Autodesk Inventor part; units mm, degrees
ref_plane "YZ Plane" through (0, 0, 0) normal (1, 0, 0) x (0, 1, 0)
ref_plane "XZ Plane" through (0, 0, 0) normal (0, 1, 0) x (-1, 0, 0)
ref_plane "XY Plane" through (0, 0, 0) normal (0, 0, 1) x (1, 0, 0)
sketch "Sketch1" plane through (0, 0, 0) normal (0, 1, 0) x (-1, 0, 0)
  line L0 (0, 0) -> (50, 0)
  line L1 (50, 0) -> (50, -70)
  line L2 (50, -70) -> (0, -70)
  line L3 (0, -70) -> (0, 0)
  dimension "d0" = 50
  dimension "d1" = 70
extrude "Extrusion1" add sketch "Sketch1" along normal blind 2
sketch "Sketch2" plane through (0, 2, 0) normal (0, 1, 0) x (1, 0, 0)
  line L0 (-47.6458, 6.5409) -> (-28.6458, 6.5409)
  line L1 (-28.6458, 6.5409) -> (-28.6458, 18.5409)
  line L2 (-28.6458, 18.5409) -> (-47.6458, 18.5409)
  line L3 (-47.6458, 18.5409) -> (-47.6458, 6.5409)
  line L4 (-47.6458, 26.8862) -> (-28.6458, 26.8862)
  line L5 (-28.6458, 26.8862) -> (-28.6458, 38.8862)
  line L6 (-28.6458, 38.8862) -> (-47.6458, 38.8862)
  line L7 (-47.6458, 38.8862) -> (-47.6458, 26.8862)
  line L8 (-47.6458, 47.2315) -> (-28.6458, 47.2315)
  line L9 (-28.6458, 47.2315) -> (-28.6458, 59.2315)
  line L10 (-28.6458, 59.2315) -> (-47.6458, 59.2315)
  line L11 (-47.6458, 59.2315) -> (-47.6458, 47.2315)
  point P0 (0, 0)
  dimension "d4" = 19
  dimension "d5" = 12
  dimension "d6" = 19
  dimension "d7" = 12
  dimension "d8" = 19
  dimension "d9" = 12
extrude "Extrusion2" add sketch "Sketch2" along normal blind 20
properties part number "temp_pcb"
Geometry check sheet. Reference: the model listing, model coordinates, mm. A direction names the side the tool comes from. Give positions to 0.01 mm unless a question says otherwise; leave off trailing zeros. Loops run counter-clockwise (first coordinate to the right, second up) from the corner with the lowest first, then second, coordinate; pieces in that order, holes last. Notation, with made-up numbers: (-3.75, 73.25) -> (37.25, 73.25) arc R22 ccw to (37.25, 80.25) -> close; hole circle Ø7 at (38.25, 71.5). An arc over 180 degrees is marked (long way). Answer in a Markdown table with one row per item. Add a question column.
1) Cross-section at C-C on x = -42. Record the boundary of the cut face in (y, z).
2) Gauge pin test, flat ends, axial feed: P1, Ø9.5, axis at y = 13, z = -53.5, coming from the -X side; P2, Ø9.5, axis at x = -38, y = 8, coming from the +Z side; P3, Ø15, axis at x = -16.5, z = -43.5, coming from the +Y side; P4, Ø10, axis at x = -19, y = 10.5, coming from the +Z side. Record the tip position at first contact, or that the pin passes through.
3) Cross-section at B-B on z = -8. Record the boundary of the cut face in (x, y), and give its area (3 significant figures).
4) Material ranges on probe 1 along Z at (x, y) = (-44, 8.25); probe 2 along Y at (x, z) = (-7, -43); probe 3 along X at (y, z) = (20.5, -58), recorded low to high. Write a range as from..to.
5) Cross-section at A-A on y = 8.5. Record the boundary of the cut face in (x, z), and give its area (3 significant figures).
6) Draft check along Z on faces 1 (the face through (-38, 12, -18.541)), 2 (the face through (-38, 12, -6.541)), 3 (the face through (-28.646, 12, -53)). Enter one of: pulls with the +Z half, pulls with the -Z half, needs draft (parallel to the pull), parting line crosses it, or undercut.
7) Cross-section at D-D on z = -66. Record the boundary of the cut face in (x, y), and give its area (3 significant figures).
8) Set-up check for faces 4 (the face through (-38, 12, -38.886)), 5 (the face through (-38, 12, -59.232)), 6 (the face through (-47.646, 12, -13)): record each of +Z, -Z, +X, -X, +Y, -Y from which the full face is reachable in a straight line by a thin tool's end or side.
Outcome:
| question | item | result |
|---|---|---|
| 1 | outline | (0, -70) -> (2, -70) -> (2, -59.23) -> (22, -59.23) -> (22, -47.23) -> (2, -47.23) -> (2, -38.89) -> (22, -38.89) -> (22, -26.89) -> (2, -26.89) -> (2, -18.54) -> (22, -18.54) -> (22, -6.54) -> (2, -6.54) -> (2, 0) -> (0, 0) -> close |
| 2 | P1 | stops at x = -47.65 |
| 2 | P2 | stops at z = -6.54 |
| 2 | P3 | stops at y = 2 |
| 2 | P4 | passes through |
| 3 | outline | (-50, 0) -> (0, 0) -> (0, 2) -> (-28.65, 2) -> (-28.65, 22) -> (-47.65, 22) -> (-47.65, 2) -> (-50, 2) -> close |
| 3 | area | 480 mm^2 |
| 4 | probe 1 | z = -59.23..-47.23, -38.89..-26.89, -18.54..-6.54 |
| 4 | probe 2 | y = 0..2 |
| 4 | probe 3 | x = -47.65..-28.65 |
| 5 | outline | (-47.65, -59.23) -> (-28.65, -59.23) -> (-28.65, -47.23) -> (-47.65, -47.23) -> close; (-47.65, -38.89) -> (-28.65, -38.89) -> (-28.65, -26.89) -> (-47.65, -26.89) -> close; (-47.65, -18.54) -> (-28.65, -18.54) -> (-28.65, -6.54) -> (-47.65, -6.54) -> close |
| 5 | area | 684 mm^2 |
| 6 | face 1 | undercut |
| 6 | face 2 | pulls with the +Z half |
| 6 | face 3 | needs draft |
| 7 | outline | (-50, 0) -> (0, 0) -> (0, 2) -> (-50, 2) -> close |
| 7 | area | 100 mm^2 |
| 8 | face 4 | +X, -X, +Y |
| 8 | face 5 | -Z, +X, -X, +Y |
| 8 | face 6 | +Z, -Z, -X, +Y |
